from build123d import *

# Parameters (mm, degrees)
SKETCH1_R           = 5
SKETCH1_R_2         = 1.75
BOSS_EXTRUDE1_DEPTH = 4.5
BOSS_EXTRUDE2_START = -4.5
BOSS_EXTRUDE2_DEPTH = 4.5
CUT_EXTRUDE3_START  = 2.2
CUT_EXTRUDE3_DEPTH  = 0.1


# Read off the part's stored shape, not the designer's step: Cut-Extrude3
with BuildPart() as part:
    # Sketch1 → Boss-Extrude1 (new body)
    # profile 1 of 3: a face of its own
    with BuildSketch(Plane.XY):
        with Locations((-11, 0)):
            Circle(SKETCH1_R)
        with Locations((-11, 0)):
            Circle(SKETCH1_R_2, mode=Mode.SUBTRACT)
    # profile 2 of 3: a face of its own
    with BuildSketch(Plane.XY):
        with Locations((11, 0)):
            Circle(SKETCH1_R)
        with Locations((11, 0)):
            Circle(SKETCH1_R_2, mode=Mode.SUBTRACT)
    # profile 3 of 3: a face of its own
    with BuildSketch(Plane.XY):
        with BuildLine():
            Line((11, 5), (-11, 5))
            ThreePointArc((-11, 5), (-7.464466094, 3.535533906), (-6, 0))
            ThreePointArc((-6, 0), (-7.464466094, -3.535533906), (-11, -5))
            Line((-11, -5), (11.000000019, -5))
            ThreePointArc((11.000000019, -5), (6, -9e-09), (11, 5))
        make_face()
    extrude(amount=BOSS_EXTRUDE1_DEPTH)

    # Sketch5 → Boss-Extrude2 (add)
    with BuildSketch(Plane.XY.offset(4.5).offset(BOSS_EXTRUDE2_START)):
        with BuildLine():
            Line((11, -5), (13.99, -5))
            Line((13.99, -5), (20.61, -1.48))
            add(Edge.make_bspline(
                [(42.27, 6), (27.826894641, 4.768168558), (24.733930665, 2.331798547), (20.61, -1.48)],
                knots=[0, 0, 0, 0, 1, 1, 1, 1], degree=3))
            Line((42.27, 6), (49.180795902, 10.03))
            Line((49.180795902, 10.03), (46.363989199, 12.87))
            add(Edge.make_bspline(
                [(0, 5), (22.856130072, 10.87555535), (46.363989199, 12.87)],
                knots=[0, 0, 0, 1, 1, 1], degree=2))
            Line((0, 5), (11, 5))
            ThreePointArc((11, 5), (16, 0), (11, -5))
        make_face()
    extrude(amount=BOSS_EXTRUDE2_DEPTH)

    # Cut-Extrude3 outline → Cut-Extrude3 (cut)
    with BuildSketch(Plane.XY.offset(CUT_EXTRUDE3_START)):
        with BuildLine():
            add(Edge.make_bspline(
                [(38.979397214, 11.642850201), (39.348659921, 11.684028726), (39.718010294, 11.724686129), (40.087448338, 11.76482241), (40.456974055, 11.804437571), (40.826587452, 11.843531609), (41.196288532, 11.882104526), (41.566077299, 11.920156321), (41.935953757, 11.957686995), (42.305917912, 11.994696547), (42.675969767, 12.031184976), (43.046109327, 12.067152283), (43.416336595, 12.102598468), (43.786651577, 12.13752353), (44.157054276, 12.17192747)],
                knots=[0.500328151, 0.500328151, 0.500328151, 0.500328151, 0.500328151, 0.500328151, 0.500328151, 0.500328151, 0.500328151, 0.500328151, 0.500328151, 0.500328151, 0.500328151, 0.500328151, 0.500328151, 0.500437892, 0.500437892, 0.500437892, 0.500437892, 0.500437892, 0.500437892, 0.500437892, 0.500437892, 0.500437892, 0.500437892, 0.500437892, 0.500437892, 0.500437892, 0.500437892, 0.500437892], degree=14))
            Line((38.979397214, 11.642850201), (42.27, 6))
            Line((42.27, 6), (46.363989199, 8.387391656))
            Line((46.363989199, 8.387391656), (44.157054276, 12.17192747))
        make_face()
    extrude(amount=CUT_EXTRUDE3_DEPTH, mode=Mode.SUBTRACT)


solid = part.part
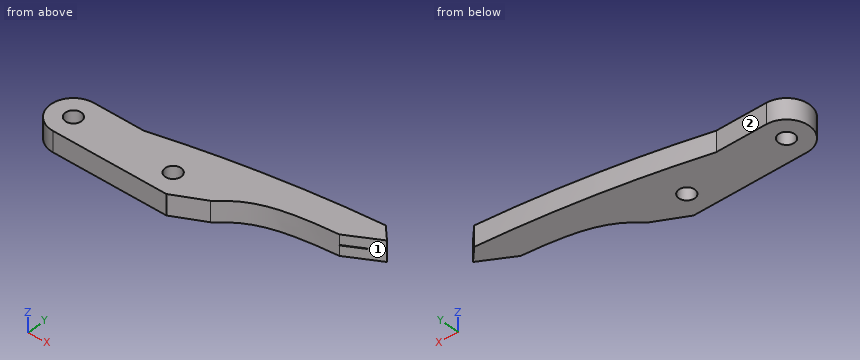
Design review of the part built by this model. Coordinates are the model's own, in mm. Face numbers are marked on the shaded views. A direction names the side the tool comes from. Coordinates: 2 decimals unless noted, no trailing zeros. Use a Markdown table: item, result. Add a question column.
Item 1: Clearance check with flat-ended pins moving along their axes: P1, Ø1.5, axis at y = 9.5, z = 3, coming from the +X side; P2, Ø3, axis at x = -11, y = 0, coming from the -Z side; P3, Ø2, axis at x = -1.5, z = 3.5, coming from the +Y side. State where each tip first meets the part, or that it passes through.
Item 2: Wall thickness on L1, parallel to Y at x = -11, z = 2.7; L2, parallel to Y at x = 11, z = 2.5; L3, parallel to Y at x = 23, z = 1.2: over which ranges is each line inside the solid? List them lowest first. Write a range as from..to.
Item 3: Machinability: for the marked faces 1 and 2, which of the approach directions +Z, -Z, +X, -X, +Y, -Y give a long, thin tool a straight path to every point of the face, cutting with its end or side? Answer none if there is none.
Item 4: We need section A-A, the plane z = 1.1. Count the separate pieces of the cut face and the enclosed holes in it, and give its area (3 significant figures).
Numbers:
| question | item | result |
|---|---|---|
| 1 | P1 | stops at x = 49.18 |
| 1 | P2 | passes through |
| 1 | P3 | stops at y = 5 |
| 2 | L1 | y = -5..-1.75, 1.75..5 |
| 2 | L2 | y = -5..-1.75, 1.75..7.59 |
| 2 | L3 | y = 0.6..9.9 |
| 3 | face 1 | +Z, -Z, +X, -Y |
| 3 | face 2 | +Z, -Z, -X, +Y |
| 4 | separate pieces | 1 |
| 4 | enclosed holes | 2 |
| 4 | area | 562 mm^2 |
